Autodesk Inventor part; units mm, degrees
sketch "Skizze1" plane through (27.583261, -56.113234, -10.899999) normal (0, 0, 1) x (1, 0, 0)
  line L0 (20.486741, 28.426785) -> (20.486741, 31.173234)
  line L1 (28.486738, 28.426785) -> (20.486741, 28.426785)
  line L2 (28.486738, 31.173234) -> (28.486738, 28.426785)
  circle A0 centre (48.116381, 27.672954) radius 3.500451
  line L3 (48.870292, 0.100002) -> (48.870292, 7.94323)
  line L4 (48.973479, 8.043232) -> (51.613555, 8.043232)
  line L5 (51.613555, 0) -> (48.973479, 0)
  circle A1 centre (48.116472, -19.586583) radius 3.50032
  line L6 (20.529933, -20.340319) -> (28.529944, -20.340319)
  line L7 (28.529944, -20.340319) -> (28.529944, -23.086762)
  line L8 (20.529933, -23.086762) -> (20.529933, -20.340319)
  circle A2 centre (0.857019, -19.586408) radius 3.500451
  line L9 (0.103188, 7.94323) -> (0.103188, 0.100002)
  line L10 (-2.640073, 8.043232) -> (0, 8.043232)
  line L11 (0, 0) -> (-2.640073, 0)
  circle A3 centre (0.856903, 27.67302) radius 3.50027
  circle A4 centre (6.691673, 3.973123) radius 1.000129
  circle A5 centre (9.236925, 3.973204) radius 1.000185
  circle A6 centre (11.781701, 3.973221) radius 0.999961
  circle A7 centre (14.326498, 3.973153) radius 0.999748
  circle A8 centre (14.3269, 0.233503) radius 0.99969
  circle A9 centre (11.78165, 0.233145) radius 1.000125
  circle A10 centre (9.236749, 0.233322) radius 0.999912
  circle A11 centre (6.691637, 0.232928) radius 1.000319
  line L12 (-2.640073, 8.043232) -> (0.103188, 8.043232)
  line L13 (0.103188, 8.043232) -> (0.103188, 0)
  line L14 (0.103188, 0) -> (-2.640073, 0)
  line L15 (20.486741, 31.173234) -> (20.486741, 28.426785)
  line L16 (28.486738, 28.426785) -> (28.486738, 31.173234)
  line L17 (48.116736, 31.173234) -> (28.486738, 31.173234)
  line L18 (0.85674, -23.086762) -> (20.529933, -23.086762)
  line L19 (-2.643261, 0.100002) -> (-2.643261, -19.586763)
  line L20 (51.616735, -19.586763) -> (51.616735, 0.100002)
  line L21 (-2.643261, 27.673233) -> (-2.643261, 7.94323)
  line L22 (20.486741, 31.173234) -> (0.85674, 31.173234)
  line L23 (51.616735, 7.94323) -> (51.616735, 27.673233)
  line L24 (28.529944, -23.086762) -> (48.116736, -23.086762)
  line L25 (-2.643261, -23.086762) -> (51.616735, -23.086762)
  line L26 (51.616735, -23.086762) -> (51.616735, 31.173234)
  line L27 (51.616735, 31.173234) -> (-2.643261, 31.173234)
  line L28 (-2.643261, 31.173234) -> (-2.643261, -23.086762)
  line L29 (51.613555, 8.043232) -> (48.870292, 8.043232)
  line L30 (48.870292, 8.043232) -> (48.870292, 0)
  line L31 (48.870292, 0) -> (51.613555, 0)
  line L32 (48.870292, 0) -> (51.613555, 0)
  line L33 (48.870292, 0) -> (48.870292, 8.043232)
  line L34 (51.613555, 8.043232) -> (48.870292, 8.043232)
  line L35 (48.870292, 8.043232) -> (48.870292, 0)
  line L36 (48.870292, 0) -> (51.613555, 0)
  line L37 (51.613555, 0) -> (51.613555, 8.043232)
  line L38 (0.103188, 0) -> (-2.640073, 0)
  line L39 (-2.640073, 8.043232) -> (0.103188, 8.043232)
  line L40 (0.103188, 0) -> (-2.640073, 0)
  line L41 (-2.640073, 0) -> (-2.640073, 8.043232)
  line L42 (-2.640073, 8.043232) -> (0.103188, 8.043232)
  line L43 (0.103188, 8.043232) -> (0.103188, 0)
  point P0 (-27.583261, 56.113234)
  point P1 (0.837182, 31.173234)
  point P2 (-2.643261, 27.700217)
  point P3 (-2.643261, -19.621008)
  point P4 (0.830931, -23.086762)
  point P5 (48.147826, -23.086762)
  point P6 (51.616735, -19.606381)
  point P7 (51.616735, 27.699042)
  point P8 (48.150981, 31.173234)
sketch "Skizze1 outline for Extrusion2" plane through (27.583261, -56.113234, -10.899999) normal (0, 0, 1) x (1, 0, 0)
  line L0 (28.486738, 28.426785) -> (20.486741, 28.426785)
  line L1 (28.486738, 31.173234) -> (28.486738, 28.426785)
  line L2 (20.486741, 28.426785) -> (20.486741, 31.173234)
  line L3 (48.116736, 31.173234) -> (28.486738, 31.173234)
  line L4 (20.486741, 31.173234) -> (0.85674, 31.173234)
  line L5 (48.150981, 31.173234) -> (48.116736, 31.173234)
  line L6 (0.85674, 31.173234) -> (0.837182, 31.173234)
  arc A0 (51.616735, 27.699042) -> (48.150981, 31.173234) centre (48.116381, 27.672954) ccw
  arc A1 (0.837182, 31.173234) -> (-2.643261, 27.700217) centre (0.856903, 27.67302) ccw
  line L7 (51.616735, 27.673233) -> (51.616735, 27.699042)
  line L8 (-2.643261, 27.700217) -> (-2.643261, 27.673233)
  line L9 (51.616735, 7.94323) -> (51.616735, 27.673233)
  line L10 (-2.643261, 27.673233) -> (-2.643261, 7.94323)
  line L11 (51.616735, 0.100002) -> (51.616735, 7.94323)
  line L12 (-2.643261, 7.94323) -> (-2.643261, 0.100002)
  line L13 (51.616735, -19.586763) -> (51.616735, 0.100002)
  line L14 (-2.643261, 0.100002) -> (-2.643261, -19.586763)
  line L15 (51.616735, -19.606381) -> (51.616735, -19.586763)
  line L16 (-2.643261, -19.586763) -> (-2.643261, -19.621008)
  arc A2 (48.147826, -23.086762) -> (51.616735, -19.606381) centre (48.116472, -19.586583) ccw
  arc A3 (-2.643261, -19.621008) -> (0.830931, -23.086762) centre (0.857019, -19.586408) ccw
  line L17 (48.116736, -23.086762) -> (48.147826, -23.086762)
  line L18 (0.830931, -23.086762) -> (0.85674, -23.086762)
  line L19 (28.529944, -23.086762) -> (48.116736, -23.086762)
  line L20 (0.85674, -23.086762) -> (20.529933, -23.086762)
  line L21 (28.529944, -20.340319) -> (28.529944, -23.086762)
  line L22 (20.529933, -23.086762) -> (20.529933, -20.340319)
  line L23 (20.529933, -20.340319) -> (28.529944, -20.340319)
  circle A4 centre (6.691637, 0.232928) radius 1.000319
  circle A5 centre (9.236749, 0.233322) radius 0.999912
  circle A6 centre (11.78165, 0.233145) radius 1.000125
  circle A7 centre (14.3269, 0.233503) radius 0.99969
  line L24 (-2.640073, 0) -> (-2.640073, 8.043232)
  line L25 (0, 0) -> (-2.640073, 0)
  line L26 (0.103188, 0) -> (0, 0)
  line L27 (0.103188, 0.100002) -> (0.103188, 0)
  line L28 (0.103188, 7.94323) -> (0.103188, 0.100002)
  line L29 (0.103188, 8.043232) -> (0.103188, 7.94323)
  line L30 (0, 8.043232) -> (0.103188, 8.043232)
  line L31 (-2.640073, 8.043232) -> (0, 8.043232)
  circle A8 centre (6.691673, 3.973123) radius 1.000129
  circle A9 centre (9.236925, 3.973204) radius 1.000185
  circle A10 centre (11.781701, 3.973221) radius 0.999961
  circle A11 centre (14.326498, 3.973153) radius 0.999748
  line L32 (51.613555, 8.043232) -> (51.613555, 0)
  line L33 (48.973479, 8.043232) -> (51.613555, 8.043232)
  line L34 (48.870292, 8.043232) -> (48.973479, 8.043232)
  line L35 (48.870292, 7.94323) -> (48.870292, 8.043232)
  line L36 (48.870292, 0.100002) -> (48.870292, 7.94323)
  line L37 (48.870292, 0) -> (48.870292, 0.100002)
  line L38 (48.973479, 0) -> (48.870292, 0)
  line L39 (51.613555, 0) -> (48.973479, 0)
extrude "Extrusion2" add sketch "Skizze1 outline for Extrusion2" along normal blind 1.8
sketch "Skizze2" plane through (27.583261, -56.113234, -9.099999) normal (0, 0, 1) x (1, 0, 0)
  line L0 (4.491739, -1.966767) -> (16.526742, -1.966767)
  line L1 (4.491739, -1.966767) -> (4.491739, 6.173234)
  line L2 (16.526742, 6.173234) -> (16.526742, -1.966767)
  line L3 (4.491739, 6.173234) -> (16.526742, 6.173234)
  line L4 (16.526742, -1.966767) -> (4.491739, -1.966767)
  circle A0 centre (9.236925, 3.973204) radius 1.000185
  circle A1 centre (11.781802, 3.973293) radius 1.000086
  circle A2 centre (14.32665, 3.9735) radius 1.00028
  circle A3 centre (14.326722, 0.233403) radius 0.999832
  circle A4 centre (11.78165, 0.233145) radius 1.000125
  circle A5 centre (9.236749, 0.233322) radius 0.999912
  circle A6 centre (6.691673, 3.973123) radius 1.000129
  circle A7 centre (6.691637, 0.232928) radius 1.000319
  point P0 (-27.583261, 56.113234)
extrude "Extrusion3" add sketch "Skizze2" along normal blind 4
sketch "Skizze3" plane through (27.583261, -56.113234, -9.099999) normal (0, 0, 1) x (1, 0, 0)
  circle A0 centre (12.321135, -8.122127) radius 2.666057
  circle A1 centre (12.321681, -8.121848) radius 3.499995
  circle A2 centre (12.3219, -8.121781) radius 2.666437
  circle A3 centre (12.321203, -8.121912) radius 3.500477
  circle A4 centre (24.486223, 4.041641) radius 4.998329
  circle A5 centre (24.486657, 4.043031) radius 2.66645
  circle A6 centre (36.651848, 16.208558) radius 2.666928
  circle A7 centre (36.651807, 16.208589) radius 3.500291
  line L0 (51.613555, 8.043232) -> (51.613555, 0)
  line L1 (51.613555, 4.021616) -> (-2.640073, 4.021616) construction
  line L2 (-2.640073, 0) -> (-2.640073, 8.043232)
  circle A8 centre (12.321135, 16.165359) radius 2.666057
  circle A9 centre (12.321203, 16.165144) radius 3.500477
  circle A10 centre (36.651848, -8.165326) radius 2.666928
  circle A11 centre (36.651807, -8.165357) radius 3.500291
  point P0 (-27.583261, 56.113234)
  point P1 (10.243668, -6.451202)
  point P2 (12.201311, -10.78549)
extrude "Extrusion4" add sketch "Skizze3" along normal blind 2
sketch "Skizze4" plane through (27.583261, -56.113234, -9.099999) normal (0, 0, 1) x (1, 0, 0)
  line L0 (51.616735, -19.606381) -> (51.616735, 27.699042) construction
  line L1 (51.616735, 4.04633) -> (-2.640073, 4.021616) construction
  line L2 (-2.640073, 0) -> (-2.640073, 8.043232) construction
  circle A0 centre (36.651848, 16.208558) radius 2.666928 construction
  circle A1 centre (36.651807, 16.208589) radius 3.500291 construction
  circle A2 centre (12.321681, -8.121848) radius 3.499995 construction
  arc A3 (12.201311, -10.78549) -> (10.243668, -6.451202) centre (12.3219, -8.121781) ccw construction
  arc A4 (10.243668, -6.451202) -> (12.201311, -10.78549) centre (12.321135, -8.122127) ccw construction
  circle A5 centre (24.486657, 4.043031) radius 2.66645 construction
  circle A6 centre (36.651848, 16.208558) radius 2.666928 construction
  arc A7 (10.243668, -6.451202) -> (12.201311, -10.78549) centre (12.321135, -8.122127) ccw construction
  arc A8 (12.201311, -10.78549) -> (10.243668, -6.451202) centre (12.3219, -8.121781) ccw construction
  point P0 (-27.583261, 56.113234)
properties part number "brick_bottom_standard"
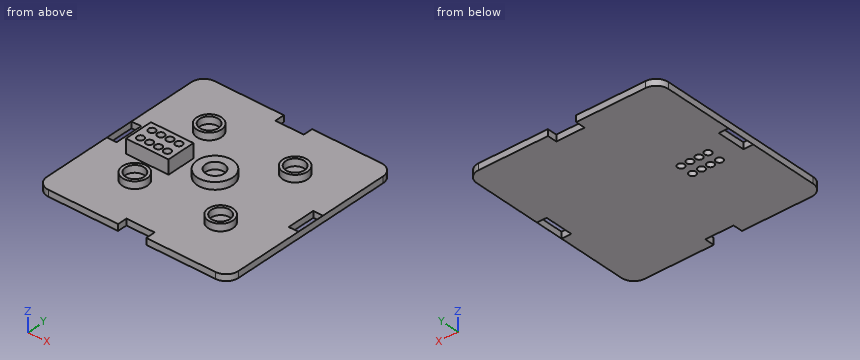
Check sheet for the modelled part. Datum: model origin and axes. Units: mm. Coordinates: 2 decimals unless noted, no trailing zeros. Write each loop counter-clockwise with the first axis right and the second up, starting at its lowest first coordinate (ties: lowest second). Pieces come first, ordered by that corner, then holes. Notation, with made-up numbers: M 54,52.5 L 61,52.5 A31 ccw 61,86.5 Z; hole C -39.5,-20 d7. An arc over 180 degrees is marked long. Answer as CSV lines item,"result".
Q1. Cross-section at C-C (y = -34). Record the boundary of the cut face in (x, z).
Check result:
outline,"M 24.94,-10.9 L 79.2,-10.9 L 79.2,-9.1 L 24.94,-9.1 Z"
Q2. Cross-section at B-B (x = 65.5). Record the boundary of the cut face in (y, z).
Check result:
outline,"M -79.2,-10.9 L -24.94,-10.9 L -24.94,-9.1 L -36.64,-9.1 L -36.64,-7.1 L -37.56,-7.1 L -37.56,-9.1 L -42.25,-9.1 L -42.25,-7.1 L -43.17,-7.1 L -43.17,-9.1 L -61.01,-9.1 L -61.01,-7.1 L -61.93,-7.1 L -61.93,-9.1 L -66.63,-9.1 L -66.63,-7.1 L -67.54,-7.1 L -67.54,-9.1 L -79.2,-9.1 Z"
Q3. Material ranges on probe 1 along Y at (x, z) = (35, -7.85); probe 2 along Y at (x, z) = (52, -8.3); probe 3 along X at (y, z) = (-65, -7.15), recorded low to high. Write a range as from..to.
Check result:
probe 1,"-58.08..-56.57, -55.19..-52.83, -51.45..-49.94"
probe 2,"-57.07..-54.74, -49.4..-47.07"
probe 3,"36.49..37.35, 42.46..43.32, 60.81..61.67, 66.8..67.66"
Q4. Cross-section at A-A (z = -8.15). Count the separate pieces of the cut face and the enclosed holes in it, then the cut area to 3 significant figures.
Check result:
separate pieces,"6"
enclosed holes,"13"
area,"194 mm^2"
Q5. Go/stop test with flat-tipped pins: pin 1 (0.9 mm diameter, centred on x = 50.5, z = -9.5, fed in from -Y); pin 2 (8 mm diameter, centred on x = 53.5, y = -51, fed in from +Z); pin 3 (0.9 mm diameter, centred on x = 52, z = -10, fed in from +Y). Record where each tip stops, or that it passes through.
Check result:
pin 1,"y = -76.45"
pin 2,"z = -7.1"
pin 3,"y = -27.69"
